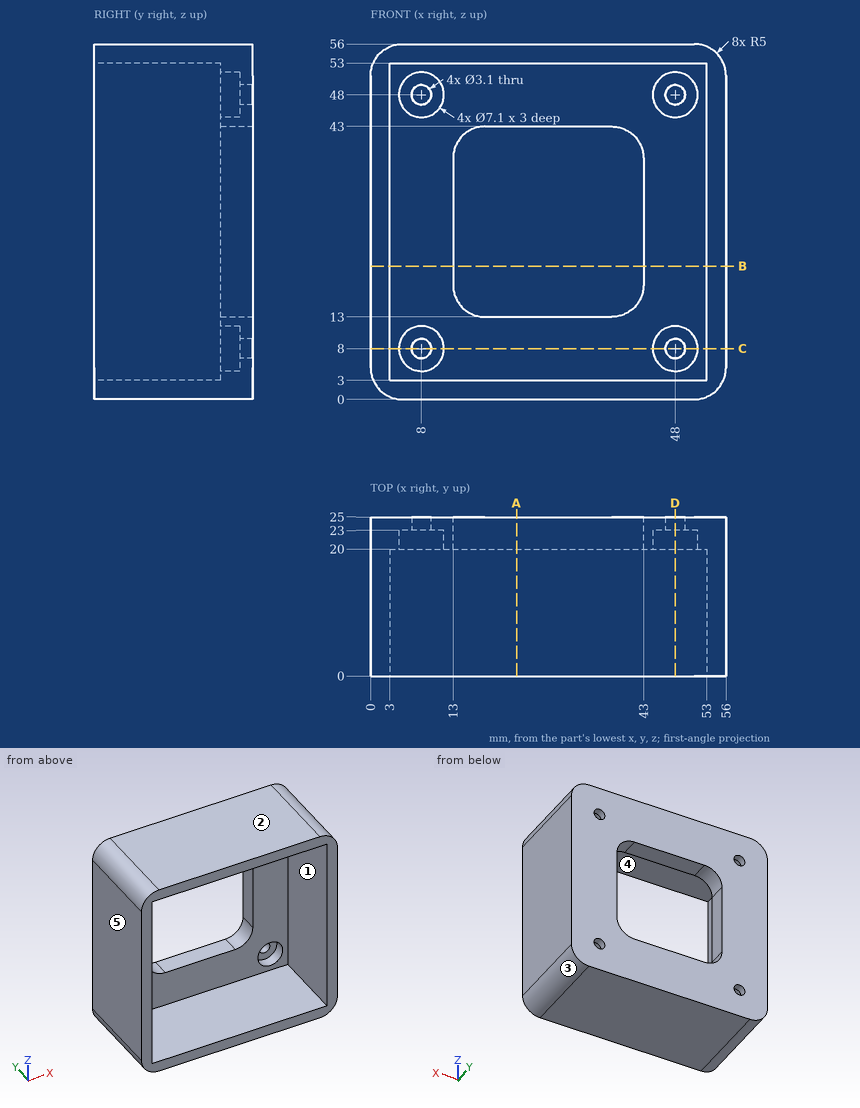
The figure shows three views and two pictorial views of one solid part (mm, origin at its lowest corner). Answer the questions. A direction names the side the tool comes from. Coordinates: 2 decimals unless noted, no trailing zeros. Write each loop counter-clockwise with the first axis right and the second up, starting at its lowest first coordinate (ties: lowest second). Pieces come first, ordered by that corner, then holes. Notation, with made-up numbers: M 69.25,38 L 85.25,38 A20 ccw 85.25,76 Z; hole C 26,57.25 d11. An arc over 180 degrees is marked long. Answer as CSV lines item,"result". Start each with the question number.
Item 1: A tool of negligible diameter and unlimited length cuts with its end or side. For the marked faces 1 and 2, from which of +Z, -Z, +X, -X, +Y, -Y can it reach the whole face along a straight path? Write none if from no direction.
Item 2: Flat-ended cylindrical pins translate along their axes: P1, Ø6, axis at x = 47.5, z = 9.5, coming from the -Y side; P2, Ø5.5, axis at x = 8, z = 48, coming from the -Y side; P3, Ø1.9, axis at x = 48, z = 48, coming from the -Y side. Find the tip coordinate at first contact, or state that the pin passes through.
Item 3: Section D-D on x = 48 is taken. Write down the section's boundary in (y, z), and give its area (3 significant figures).
Item 4: Section B-B on z = 21 is taken. Write down the section's boundary in (x, y).
Item 5: Consider L1, parallel to X at y = 24, z = 48; L2, parallel to Z at x = 8, y = 21.3; L3, parallel to X at y = 6, z = 47.5. Determine where each line is inside the solid, lowest interval first.
Item 6: Section A-A on x = 23 is taken. Write down the section's boundary in (y, z), and give its area (3 significant figures).
Item 7: Section C-C on z = 8 is taken. Write down the section's boundary in (x, y).
Item 8: Determine the mould class of the marked faces 3, 4 and 5 for opening direction Z: released by +Z, released by -Z, zero draft, split by the parting line, or undercut.
Checks:
1,face 1,"-Y"
1,face 2,"+Z, +X, -X, +Y, -Y"
2,P1,"stops at y = 20"
2,P2,"stops at y = 23"
2,P3,"passes through"
3,outline,"M 0,0 L 25,0 L 25,6.45 L 23,6.45 L 23,4.45 L 20,4.45 L 20,3 L 0,3 Z; M 0,53 L 20,53 L 20,51.55 L 23,51.55 L 23,49.55 L 25,49.55 L 25,56 L 0,56 Z; M 20,11.55 L 23,11.55 L 23,9.55 L 25,9.55 L 25,46.45 L 23,46.45 L 23,44.45 L 20,44.45 Z"
3,area,"345 mm²"
4,outline,"M 0,0 L 3,0 L 3,20 L 13,20 L 13,25 L 0,25 Z; M 43,20 L 53,20 L 53,0 L 56,0 L 56,25 L 43,25 Z"
5,L1,"x = 0 to 6.45, 9.55 to 46.45, 49.55 to 56"
5,L2,"z = 0 to 4.45, 11.55 to 44.45, 51.55 to 56"
5,L3,"x = 0 to 3, 53 to 56"
6,outline,"M 0,0 L 25,0 L 25,13 L 20,13 L 20,3 L 0,3 Z; M 0,53 L 20,53 L 20,43 L 25,43 L 25,56 L 0,56 Z"
6,area,"250 mm²"
7,outline,"M 0,0 L 3,0 L 3,20 L 4.45,20 L 4.45,23 L 6.45,23 L 6.45,25 L 0,25 Z; M 9.55,23 L 11.55,23 L 11.55,20 L 44.45,20 L 44.45,23 L 46.45,23 L 46.45,25 L 9.55,25 Z; M 49.55,23 L 51.55,23 L 51.55,20 L 53,20 L 53,0 L 56,0 L 56,25 L 49.55,25 Z"
8,face 3,"released by -Z"
8,face 4,"undercut"
8,face 5,"zero draft"
